Check sheet for the modelled part. Datum: model origin and axes. Units: mm. A direction names the side the tool comes from. Give positions to 0.01 mm unless a question says otherwise; leave off trailing zeros. Write each loop counter-clockwise with the first axis right and the second up, starting at its lowest first coordinate (ties: lowest second). Pieces come first, ordered by that corner, then holes. Notation, with made-up numbers: (-20.5, 7.25) -> (-13.5, 7.25) arc R16 cw to (-13.5, 11.25) -> close; hole circle Ø7 at (44.5, 82). An arc over 180 degrees is marked (long way). Return JSON: item names as keys, results as strings.
from build123d import *

# Parameters (mm, degrees)
F0_R        = 12.5
F1_DEPTH    = 165
F2_R        = 5
F5_DEPTH    = 120
F6_R        = 6
F7_DEPTH    = 18.501
F8_T2_ANGLE = 240.7472216417
F8_T4_ANGLE = 240.7472216417


# Not quite as in the source:
# - a fillet or chamfer that OpenCascade refuses, or shapes differently, is made with other operations: its cross-section is extruded or revolved along the edge and cut away or added


with BuildPart() as f1:
    # F0 (on Right) → F1 (new body)
    with BuildSketch(Plane.YZ):
        with Locations((0, 79.4712570496)):
            Circle(F0_R)
    extrude(amount=-F1_DEPTH)

    # F2
    f2_edges = [f1.edges().sort_by_distance(p)[0] for p in [
        (-165, -12.5, 79.471257),
    ]]
    fillet(f2_edges, radius=F2_R)

    # F4 (on face) → F5 (join)
    with BuildSketch(Plane.YZ):
        with BuildLine():
            ThreePointArc((6, 90.4371131493), (0, 91.9712570496), (-6, 90.4371131493))
            Line((-6, 90.4371131493), (-6, 68.5054009499))
            ThreePointArc((-6, 68.5054009499), (0, 66.9712570496), (6, 68.5054009499))
            Line((6, 68.5054009499), (6, 90.4371131493))
        make_face()
    extrude(amount=F5_DEPTH)

    # F6 (on face) → F7 (cut, through all)
    with BuildSketch(Plane.XZ.offset(6)):
        with Locations((110, 79.4712570496)):
            Circle(F6_R)
    extrude(amount=-F7_DEPTH, mode=Mode.SUBTRACT)

    # F8: fillet of radius 8 on 2 edges, made by hand

    # F8_s1 → F8_t2 (revolve, cut)
    with BuildSketch(Plane(origin=(0, 34.6682356906, 59.1529818038), x_dir=(1, 0, 0), z_dir=(0, 0.5056364556, 0.8627466458))):
        with BuildLine():
            ThreePointArc((112, -52.6835647356), (117.6568542495, -50.3404189851), (120, -44.6835647356))
            Line((120, -44.6835647356), (120, -52.6835647356))
            Line((120, -52.6835647356), (112, -52.6835647356))
        make_face()
    revolve(axis=Axis((120, 0, 79.4712570496), (1, 0, 0)), revolution_arc=F8_T2_ANGLE, mode=Mode.SUBTRACT)

    # F8_s3 → F8_t4 (revolve, cut)
    with BuildSketch(Plane(origin=(0, 34.6682356906, 59.1529818038), x_dir=(1, 0, 0), z_dir=(0, -0.5056364556, -0.8627466458))):
        with BuildLine():
            ThreePointArc((112, 27.6835647356), (117.6568542495, 30.0267104861), (120, 35.6835647356))
            Line((120, 35.6835647356), (120, 27.6835647356))
            Line((120, 27.6835647356), (112, 27.6835647356))
        make_face()
    revolve(axis=Axis((120, 0, 79.4712570496), (1, 0, 0)), revolution_arc=F8_T4_ANGLE, mode=Mode.SUBTRACT)


solid = f1.part
(1) Cross-section at B-B on x = -73. Enter the section's corners in (y, z).
Reply:
{"outline": "circle Ø25 at (0, 79.47)"}
(2) Release check for a two-part mould opening along X. For faces 1 (the flat face through (0, 8, 80)), 2 (the cylindrical face through (104.006, -0.084, 79.735)), 3 (the flat face through (59, 6, 79)) record: pulls with the +X half, pulls with the -X half, needs draft (parallel to the pull), parting line crosses it, or undercut.
Reply:
{"face 1": "pulls with the +X half", "face 2": "undercut", "face 3": "needs draft"}
(3) Thickness scan on L1, parallel to Y at x = 61, z = 71.75; L2, parallel to Z at x = 110, y = 1.75; L3, parallel to Z at x = 110, y = 3.25. Record the ranges inside material, lowest first.
Reply:
{"L1": "-6 to 6", "L2": "67.09 to 73.47, 85.47 to 91.85", "L3": "67.4 to 73.47, 85.47 to 91.54"}
(4) Cross-section at A-A on x = 9.5. Enter the section's corners in (y, z), then the cut area to 3 significant figures.
Reply:
{"outline": "(-6, 68.51) arc R12.5 ccw to (6, 68.51) -> (6, 90.44) arc R12.5 ccw to (-6, 90.44) -> close", "area": "288 mm^2"}
(5) Depth check by flat-ended pin: pin 1 Ø5 at (x, y) = (-16.5, -3) entering from +Z; pin 2 Ø6 at (y, z) = (-5, 75) entering from +X; pin 3 Ø7 at (y, z) = (-8.5, 75.5) entering from +X; pin 4 Ø10 at (x, y) = (54, -7) entering from +Z. Enter the tip coordinate at first touch or a pass-through.
Reply:
{"pin 1": "z = 91.96", "pin 2": "x = 120", "pin 3": "x = 119.88", "pin 4": "z = 91.81"}
(6) Set-up check for faces 4 (the flat face through (59, -6, 80)), 5 (the flat face through (-165, 0, 80)): record each of +Z, -Z, +X, -X, +Y, -Y from which the full face is reachable in a straight line by a thin tool's end or side.
Reply:
{"face 4": "+Z, -Z, +X, -Y", "face 5": "+Z, -Z, -X, +Y, -Y"}
